```python
from build123d import *

# Parameters (mm, degrees)
F0_R     = 6.35
F1_DEPTH = 38.1
F2_W     = 76.2
F2_H     = 25.4
F3_DEPTH = 12.7
F4_DEPTH = 76.2
F6_DEPTH = 12.7


with BuildPart() as f1:
    # F0 (on Top) → F1 (new body)
    with BuildSketch(Plane.XY):
        with BuildLine():
            ThreePointArc((25.4, 12.7), (21.6802561211, 21.6802561211), (12.7, 25.4))
            ThreePointArc((12.7, 25.4), (3.7197438789, 21.6802561211), (0, 12.7))
            ThreePointArc((0, 12.7), (3.7197438961, 3.7197438617), (12.7000000487, 0))
            ThreePointArc((12.7000000487, 0), (21.6802561383, 3.7197438961), (25.4, 12.7))
        make_face()
        with Locations((12.7, 12.7)):
            Circle(F0_R, mode=Mode.SUBTRACT)
    extrude(amount=F1_DEPTH)

    # F2 (on Top) → F3 (join)
    with BuildSketch(Plane.XY):
        with Locations((38.1, 12.7)):
            Rectangle(F2_W, F2_H)
    extrude(amount=F3_DEPTH)

    # F4 (cut): faces of the model
    f4_faces = [f1.faces().sort_by_distance(p)[0] for p in [
        (2.8367728246, 22.5632271754, 12.7),
        (2.8367728246, 2.8367728246, 12.7),
        (12.7, 12.7, 12.7),
    ]]
    extrude(f4_faces, amount=-F4_DEPTH, mode=Mode.SUBTRACT)

    # F5 (on face) → F6 (cut)
    with BuildSketch(Plane.XY.offset(12.7)):
        with BuildLine():
            ThreePointArc((38.1, 19.05), (42.5901280605, 17.1901280605), (44.45, 12.7))
            ThreePointArc((44.45, 12.7), (42.5901280605, 8.2098719395), (38.1, 6.35))
            Line((38.1, 6.35), (59.7659657613, 6.35))
            ThreePointArc((59.7659657613, 6.35), (53.4159657613, 12.7), (59.7659657613, 19.05))
            Line((59.7659657613, 19.05), (38.1, 19.05))
        make_face()
        with BuildLine():
            ThreePointArc((38.1, 6.35), (42.5901280605, 8.2098719395), (44.45, 12.7))
            ThreePointArc((44.45, 12.7), (42.5901280605, 17.1901280605), (38.1, 19.05))
            ThreePointArc((38.1, 19.05), (31.75, 12.7), (38.1, 6.35))
        make_face()
        with BuildLine():
            ThreePointArc((66.1159657613, 12.7), (64.2560938218, 17.1901280605), (59.7659657613, 19.05))
            ThreePointArc((59.7659657613, 19.05), (53.4159657613, 12.7), (59.7659657613, 6.35))
            ThreePointArc((59.7659657613, 6.35), (64.2560938218, 8.2098719395), (66.1159657613, 12.7))
        make_face()
        with BuildLine():
            ThreePointArc((66.8432824171, 25.4), (72.9122904211, 21.7280036784), (76.2, 15.4425139708))
            Line((76.2, 15.4425139708), (76.2, 25.4))
            Line((76.2, 25.4), (66.8432824171, 25.4))
        make_face()
        with BuildLine():
            ThreePointArc((76.2, 9.9574860292), (72.9122904211, 3.6719963216), (66.8432824171, 0))
            Line((66.8432824171, 0), (76.2, 0))
            Line((76.2, 0), (76.2, 9.9574860292))
        make_face()
    extrude(amount=-F6_DEPTH, mode=Mode.SUBTRACT)


solid = f1.part
```
The model under review builds one solid part; all positions refer to its coordinate system, in mm. A direction names the side the tool comes from. Give positions to 0.01 mm unless a question says otherwise; leave off trailing zeros. Loops run counter-clockwise (first coordinate to the right, second up) from the corner with the lowest first, then second, coordinate; pieces in that order, holes last. Notation, with made-up numbers: (-4, -22) - (0, -22) arc R24 cw to (0, 16) - close; hole circle Ø11 at (86.5, 76.5). An arc over 180 degrees is marked (long way). Answer as a JSON object with one key per item and string values.
Q1. Add section B-B on x = 17. State the section outline as (y, z) points.
Worked out:
{"outline": "(0, 0) - (8.03, 0) - (8.03, 38.1) - (0.75, 38.1) - (0.75, 12.7) - (0, 12.7) - close; (17.37, 0) - (25.4, 0) - (25.4, 12.7) - (24.65, 12.7) - (24.65, 38.1) - (17.37, 38.1) - close"}
Q2. Insertion check: pin 1 (3 mm diameter, centred on y = 7, z = 5, fed in from +X); pin 2 (12.5 mm diameter, centred on x = 45, y = 13, fed in from +Z); pin 3 (1 mm diameter, centred on y = 8, z = 16, fed in from -X). Each pin has a flat end and moves straight along its axis. Give the tip position at first contact, or say it passes through.
Worked out:
{"pin 1": "stops at x = 75.8", "pin 2": "stops at z = 12.7", "pin 3": "stops at x = 0.71"}
Q3. To check wall thickness, follow line 1 along X through (y, z) = (12.7, 4.75); line 2 along X through (y, z) = (12.7, 18.5); line 3 along Y through (x, z) = (65.5, 2.5). State the ranges of each line that lie inside material, in increasing order.
Worked out:
{"line 1": "x = 0 to 6.35, 19.05 to 31.75, 66.12 to 76.2", "line 2": "x = 0 to 6.35, 19.05 to 25.4", "line 3": "y = 0 to 9.97, 15.43 to 25.4"}
Q4. Mouldability with a two-part tool opening along X and no side actions: class faces 3 (the cylindrical face through (72.981, 3.746, 6.439)), 4 (the cylindrical face through (31.75, 12.84, 6.44)), 5 (the flat face through (39, 0, 6)), 6 (the flat face through (49, 6.35, 6)) as +X half, -X half, draft (parallel to the pull), parting line (faces both ways), or undercut.
Worked out:
{"face 3": "+X half", "face 4": "undercut", "face 5": "draft", "face 6": "undercut"}
Q5. For faces 1 (the flat face through (49, 19.05, 6)), 2 (the flat face through (15, 19, 38.1)), list the 3-axis set-ups (+Z, -Z, +X, -X, +Y, -Y) from which the entire face can be reached by the end or side of a thin tool; tool diameter is ignored.
Worked out:
{"face 1": "+Z, -Z", "face 2": "+Z, +X, -X, +Y, -Y"}
Q6. Add section D-D on y = 17.5. State the section outline as (x, z) points, plus the area to 3 significant figures.
Worked out:
{"outline": "(0.94, 0) - (8.54, 0) - (8.54, 38.1) - (0.94, 38.1) - close; (16.86, 0) - (33.94, 0) - (33.94, 12.7) - (24.46, 12.7) - (24.46, 38.1) - (16.86, 38.1) - close; (63.92, 0) - (75.58, 0) - (75.58, 12.7) - (63.92, 12.7) - close", "area": "848 mm^2"}
Q7. Add section A-A on z = 11. State the section outline as (x, y) points, plus the area to 3 significant figures.
Worked out:
{"outline": "(12.7, 0) - (66.84, 0) arc R13.18 ccw to (76.2, 9.96) - (76.2, 15.44) arc R13.18 ccw to (66.84, 25.4) - (12.7, 25.4) arc R12.7 ccw to start; hole circle Ø12.7 at (12.7, 12.7); hole (38.1, 6.35) - (59.77, 6.35) arc R6.35 ccw to (59.77, 19.05) - (38.1, 19.05) arc R6.35 ccw to start", "area": "1,280 mm^2"}
Q8. Add section C-C on y = 8. State the section outline as (x, z) points.
Worked out:
{"outline": "(0.9, 0) - (8.43, 0) - (8.43, 38.1) - (0.9, 38.1) - close; (16.97, 0) - (33.83, 0) - (33.83, 12.7) - (24.5, 12.7) - (24.5, 38.1) - (16.97, 38.1) - close; (64.04, 0) - (75.62, 0) - (75.62, 12.7) - (64.04, 12.7) - close"}
